The model under review builds one solid part; all positions refer to its coordinate system, in mm. Round coordinates to 2 decimals unless told otherwise and drop trailing zeros. Write each loop counter-clockwise with the first axis right and the second up, starting at its lowest first coordinate (ties: lowest second). Pieces come first, ordered by that corner, then holes.
Item 1: Draft analysis for pull direction Y (two halves, no side actions). For faces 1 (the face through (35, -36.1, 14)), 2 (the face through (0, 1, 24)), 3 (the face through (32.182, -19.243, 0.847)), 4 (the face through (35.67, 37.74, 59.98)), state which applies: +Y half, -Y half, draft (parallel to the pull), parting line (faces both ways), or undercut.
Item 2: Add section C-C (x = 25). Give the boundary of the cut face in (y, z), plus the area to 3 significant figures.
Item 3: Add section A-A (z = 0). Give the boundary of the cut face in (x, y), plus the area to 3 significant figures.
Item 4: Add section B-B (y = 0). Give the boundary of the cut face in (x, z), plus the area to 3 significant figures.
Item 5: To check wall thickness, follow L1, parallel to Z at x = 46, y = 0; L2, parallel to Z at x = 31, y = -1; L3, parallel to Y at x = 13.5, z = -12. State the ranges of each line that lie inside material, in increasing order.
```python
from build123d import *

# Parameters (mm, degrees)
F0_W     = 75.365622
F0_H     = 88.876544
F0_R     = 19.261813
F1_DEPTH = 70.358
F2_R     = 5.08


with BuildPart() as f1:
    # F0 (on Right) → F1 (new body)
    with BuildSketch(Plane.YZ):
        with Locations((1.58331, 16.994209)):
            Rectangle(F0_W, F0_H)
        Circle(F0_R, mode=Mode.SUBTRACT)
    extrude(amount=F1_DEPTH)

    # F2
    f2_edges = [f1.edges().sort_by_distance(p)[0] for p in [
        (35.179, -36.099501, 61.432481),
        (35.179, 39.266121, 61.432481),
        (70.358, 1.58331, 61.432481),
        (0, 1.58331, 61.432481),
        (70.358, -19.261813, 0),
    ]]
    fillet(f2_edges, radius=F2_R)


solid = f1.part
```
Numbers:
1. face 1: -Y half
1. face 2: draft
1. face 3: undercut
1. face 4: +Y half
2. outline: (-36.1, -27.44) - (39.27, -27.44) - (39.27, 56.35) arc R5.08 ccw to (34.19, 61.43) - (-31.02, 61.43) arc R5.08 ccw to (-36.1, 56.35) - close; hole circle Ø38.52 at (0, 0)
2. area: 5,520 mm2
3. outline: (0, -36.1) - (70.36, -36.1) - (70.36, -24.34) arc R5.08 ccw to (65.28, -19.26) - (0, -19.26) - close; (0, 19.26) - (65.28, 19.26) arc R5.08 ccw to (70.36, 24.34) - (70.36, 39.27) - (0, 39.27) - close
3. area: 2,580 mm2
4. outline: (0, -27.44) - (70.36, -27.44) - (70.36, -24.34) arc R5.08 ccw to (65.28, -19.26) - (0, -19.26) - close; (0, 19.26) - (65.28, 19.26) arc R5.08 ccw to (70.36, 24.34) - (70.36, 56.35) arc R5.08 ccw to (65.28, 61.43) - (5.08, 61.43) arc R5.08 ccw to (0, 56.35) - close
4. area: 3,520 mm2
5. L1: z = -27.44 to -19.26, 19.26 to 61.43
5. L2: z = -27.44 to -19.24, 19.24 to 61.43
5. L3: y = -36.1 to -15.07, 15.07 to 39.27
